Here's how the part is built. I have some questions about the finished solid (model axes, mm). A direction names the side the tool comes from. Round coordinates to 2 decimals unless told otherwise and drop trailing zeros. Write each loop counter-clockwise with the first axis right and the second up, starting at its lowest first coordinate (ties: lowest second). Pieces come first, ordered by that corner, then holes. Notation, with made-up numbers: (79.5, 50) - (115.5, 50) arc R18 cw to (115.5, 71) - close; hole circle Ø10 at (2.25, -33.75). An arc over 180 degrees is marked (long way). One line per item, written item: value. Start each with the question number.
Item 1: For P1, Ø5.5, axis at x = -6, y = -35.09, coming from the -Z side; P2, Ø12, axis at y = 3, z = -118, coming from the -X side; P3, Ø1.3, axis at x = -1.5, z = -89.5, coming from the +Y side; P4, Ø3.5, axis at x = -3, z = -78.5, coming from the -Y side, each with a flat end and sliding along its axis, tell me the tip position at first contact or that it passes through.
Item 2: Imagine slicing it at D-D, the plane y = -21.5. Please give me the cut outline in (x, z), then the cut area to 3 significant figures.
Item 3: Imagine slicing it at C-C, the plane y = -8. Please give me the cut outline in (x, z).
Item 4: Imagine slicing it at A-A, the plane z = -145.5. Please give me the cut outline in (x, y) (3 decimals), then the cut area to 3 significant figures.
Item 5: Thinking about a two-plate mould opening in Z: for faces 1 (the face through (0, 0, -81)), 2 (the face through (-1, 3, 0)), 3 (the face through (-1, 3, -164)), 4 (the face through (-3, 32, -138.396)), which applies, released by +Z, released by -Z, zero draft, split by the parting line, or undercut?
Item 6: For faces 5 (the face through (-2.393, -23.758, -83.148)), 6 (the face through (-2, 26.802, -81)), 7 (the face through (-2, -26.802, -81)), which set-ups out of +Z, -Z, +X, -X, +Y, -Y let a thin tool reach every point of the face, with its end or its side?
Item 7: If I drill on line 1 (Y direction, x = -4.75, z = -7); line 2 (Y direction, x = -6, z = -150.5) (3 decimals); line 3 (Y direction, x = -2.5, z = -15), over which ranges is the centre line in solid material (lowest first)?
Item 8: Imagine slicing it at B-B, the plane z = -92.5. Please give me the cut outline in (x, y), then the cut area to 3 significant figures.
```python
from build123d import *

# Parameters (mm, degrees)
CROQUIS1_R              = 3.175
SALIENTE_EXTRUIR1_DEPTH = 164
REDONDEO1_R             = 10
CROQUIS3_W              = 112.791812306
CROQUIS3_H              = 18.145434914
CORTAR_EXTRUIR2_DEPTH   = 13


with BuildPart() as part:
    # Croquis1 → Saliente-Extruir1 (new body)
    with BuildSketch(Plane.XY):
        with BuildLine():
            Line((-1.6, 25.646228096), (-8.98691391, 29.886314259))
            ThreePointArc((-8.98691391, 29.886314259), (-9.006535925, 40.28237342), (0, 35.09))
            Line((0, 35.09), (0, -35.09))
            ThreePointArc((0, -35.09), (-9.006535925, -40.28237342), (-8.98691391, -29.886314259))
            Line((-8.98691391, -29.886314259), (-1.6, -25.646228096))
            Line((-1.6, -25.646228096), (-1.6, 25.646228096))
        make_face()
        with Locations((-6, 35.09)):
            Circle(CROQUIS1_R, mode=Mode.SUBTRACT)
        with Locations((-6, -35.09)):
            Circle(CROQUIS1_R, mode=Mode.SUBTRACT)
    extrude(amount=-SALIENTE_EXTRUIR1_DEPTH)

    # Redondeo1
    redondeo1_edges = [part.edges().sort_by_distance(p)[0] for p in [
        (-1.6, -25.646228096, -82),
        (-1.6, 25.646228096, -82),
    ]]
    fillet(redondeo1_edges, radius=REDONDEO1_R)

    # Croquis3 → Cortar-Extruir2 (cut, through all)
    with BuildSketch(Plane(origin=(0, 0, 0), x_dir=(0, 0, -1), z_dir=(1, 0, 0))):
        with Locations((82, 35.875128035)):
            Rectangle(CROQUIS3_W, CROQUIS3_H)
        with Locations((82, -35.875128035)):
            Rectangle(CROQUIS3_W, CROQUIS3_H)
    extrude(amount=-CORTAR_EXTRUIR2_DEPTH, mode=Mode.SUBTRACT)


solid = part.part
```
Values follow:
1. P1: passes through
1. P2: stops at x = -1.6
1. P3: stops at y = 26.8
1. P4: stops at y = -26.8
2. outline: (-1.74, -164) - (0, -164) - (0, 0) - (-1.74, 0) - close
2. area: 285 mm^2
3. outline: (-1.6, -164) - (0, -164) - (0, 0) - (-1.6, 0) - close
4. outline: (-8.987, -29.886) arc R6 ccw (long way) to (0, -35.09) - (0, 35.09) arc R6 ccw (long way) to (-8.987, 29.886) - (-6.622, 28.529) arc R10 cw to (-1.6, 19.856) - (-1.6, -19.856) arc R10 cw to (-6.622, -28.529) - close; hole circle Ø6.35 at (-6, -35.09); hole circle Ø6.35 at (-6, 35.09)
4. area: 303 mm^2
5. face 1: zero draft
5. face 2: released by +Z
5. face 3: released by -Z
5. face 4: undercut
6. face 5: +Z, -Z, -X
6. face 6: +X, -X, +Y
6. face 7: +X, -X, -Y
7. line 1: y = -40.96 to -38.01, -32.17 to -27.14, 27.14 to 32.17, 38.01 to 40.96
7. line 2: y = -41.09 to -38.265, -31.915 to -28.141, 28.141 to 31.915, 38.265 to 41.09
7. line 3: y = -39.96 to -24, 24 to 39.96
8. outline: (-4.41, -26.8) - (0, -26.8) - (0, 26.8) - (-4.41, 26.8) arc R10 cw to (-1.6, 19.86) - (-1.6, -19.86) arc R10 cw to start
8. area: 97.9 mm^2
